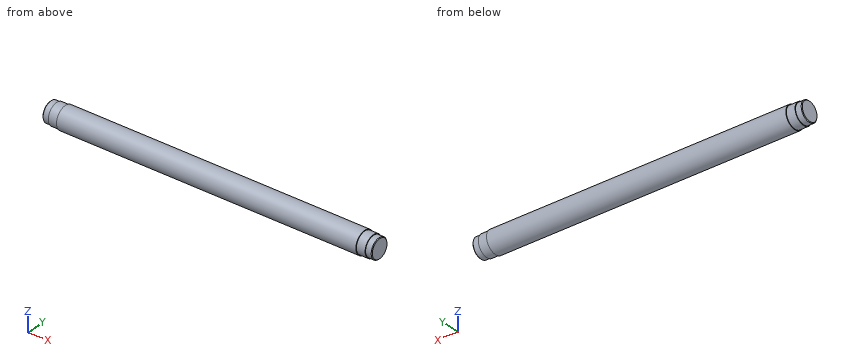
from build123d import *

# Parameters (mm, degrees)
CHAMFER_1_SIZE = 0.5
CHAMFER_2_SIZE = 0.5


with BuildPart() as part:
    # 草图1 → 旋转1 (revolve)
    with BuildSketch(Plane(origin=(0, 0, 0), x_dir=(1, 0, 0), z_dir=(0, 1, 0)), mode=Mode.PRIVATE) as revolve_1_sk:
        Polygon((0, 0), (0, 8), (5, 8), (5, 8.5), (12, 8.5), (12, 9), (252, 9), (252, 8.5), (259, 8.5), (259, 8), (264, 8), (264, 0), align=None)
    revolve(revolve_1_sk.sketch.rotate(Axis((-102.487167665, 0, 0), (1, 0, 0)), 180), axis=Axis((-102.487167665, 0, 0), (1, 0, 0)))

    # 倒角1
    chamfer_1_edges = [part.edges().sort_by_distance(p)[0] for p in [
        (264, 0, -8),
    ]]
    chamfer(chamfer_1_edges, length=CHAMFER_1_SIZE)

    # 倒角2
    chamfer_2_edges = [part.edges().sort_by_distance(p)[0] for p in [
        (0, 0, -8),
    ]]
    chamfer(chamfer_2_edges, length=CHAMFER_2_SIZE)


solid = part.part
Can you work these out from the model? Positions are in its coordinate system, mm. Coordinates: 2 decimals unless noted, no trailing zeros. Order: outer loops, then holes, each group sorted by start corner. A loop starts at its lowest first (then second) coordinate and runs counter-clockwise, first axis right, second up. Notation, with made-up numbers: (3.25, 31) - (54.25, 31) arc R17 cw to (54.25, 63) - close; hole circle Ø7 at (-5, 26.25). An arc over 180 degrees is marked (long way). Answer as a JSON object with one key per item and string values. Group by question number.
Q1. I need wall thicknesses on line 1 (Y direction, x = 100, z = 0.75); line 2 (X direction, y = 7, z = 4); line 3 (Z direction, x = 185, y = 0.25). Which ranges of each line are inside material? Lowest first, please. Write a range as from..to.
Q2. Imagine slicing it at A-A (x = 133.5). Please give me the cut outline in (y, z).
Q3. Will these pins go through, and if not, where does the flat tip stop? P1, Ø5, axis at x = 187, z = 5, coming from the +Y side; P2, Ø1.5, axis at x = 38.5, y = 7, coming from the +Z side; P3, Ø1.5, axis at x = 121.5, y = 3.5, coming from the +Z side.
Determined:
{
 "1": {"line 1": "y = -8.97..8.97", "line 2": "x = 5..259", "line 3": "z = -9..9"},
 "2": {"outline": "circle Ø18 at (0, 0)"},
 "3": {"P1": "stops at y = 8.65", "P2": "stops at z = 6.48", "P3": "stops at z = 8.57"}
}
